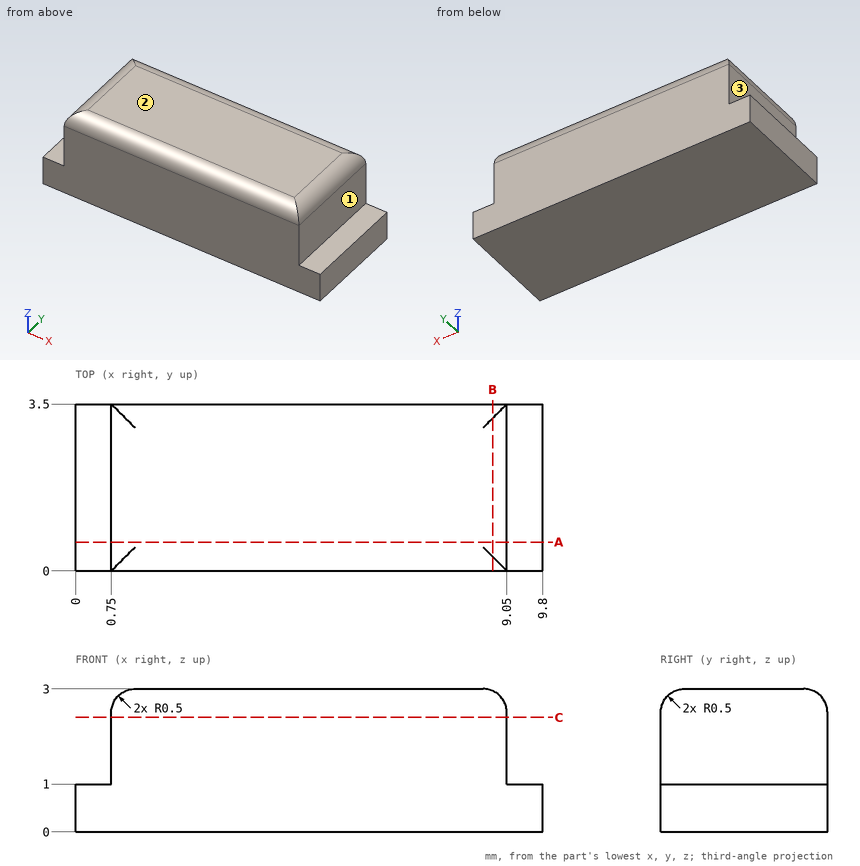
For this review, use the dimensioned drawing (mm, ordinates from the lowest corner) and the shaded views. A direction names the side the tool comes from. Give positions to 0.01 mm unless a question says otherwise; leave off trailing zeros. Order: outer loops, then holes, each group sorted by start corner. A loop starts at its lowest first (then second) coordinate and runs counter-clockwise, first axis right, second up. Notation, with made-up numbers: (-8.5, -3.5) - (31.5, -3.5) arc R20 cw to (31.5, 24.5) - close; hole circle Ø3 at (73.25, 44). An arc over 180 degrees is marked (long way). Use CSV: the item, a comma, the result in double quotes. Start each with the question number.
Q1. Take a section at B-B (x = 8.75). State the section outline as (y, z) points, and give its area (3 significant figures).
Q2. For line 1 (X direction, y = 2.5, z = 2.4); line 2 (Z direction, x = 7, y = 0.45); line 3 (Z direction, x = 8.5, y = 3.35), list the stretches that pass through material, from the lowest coordinate up.
Q3. For P1, Ø0.8, axis at y = 2, z = 2, coming from the -X side, flat-tipped, find the tip position at first contact; note if it passes through.
Q4. Machinability: for the marked faces 1, 2 and 3, which of the approach directions +Z, -Z, +X, -X, +Y, -Y give a long, thin tool a straight path to every point of the face, cutting with its end or side? Answer none if there is none.
Q5. Take a section at A-A (y = 0.6). State the section outline as (x, z) points.
Q6. Take a section at C-C (z = 2.4). State the section outline as (x, y) points.
Calculated:
1,outline,"(0, 0) - (3.5, 0) - (3.5, 2.5) arc R0.5 ccw to (3.2, 2.96) - (0.3, 2.96) arc R0.5 ccw to (0, 2.5) - close"
1,area,"10.3 mm²"
2,line 1,"x = 0.75 to 9.05"
2,line 2,"z = 0 to 3"
2,line 3,"z = 0 to 2.86"
3,P1,"stops at x = 0.75"
4,face 1,"+Z, +X, +Y, -Y"
4,face 2,"+Z, +X, -X, +Y, -Y"
4,face 3,"+Z, -X, +Y, -Y"
5,outline,"(0, 0) - (9.8, 0) - (9.8, 1) - (9.05, 1) - (9.05, 2.5) arc R0.5 ccw to (8.55, 3) - (1.25, 3) arc R0.5 ccw to (0.75, 2.5) - (0.75, 1) - (0, 1) - close"
6,outline,"(0.75, 0) - (9.05, 0) - (9.05, 3.5) - (0.75, 3.5) - close"
